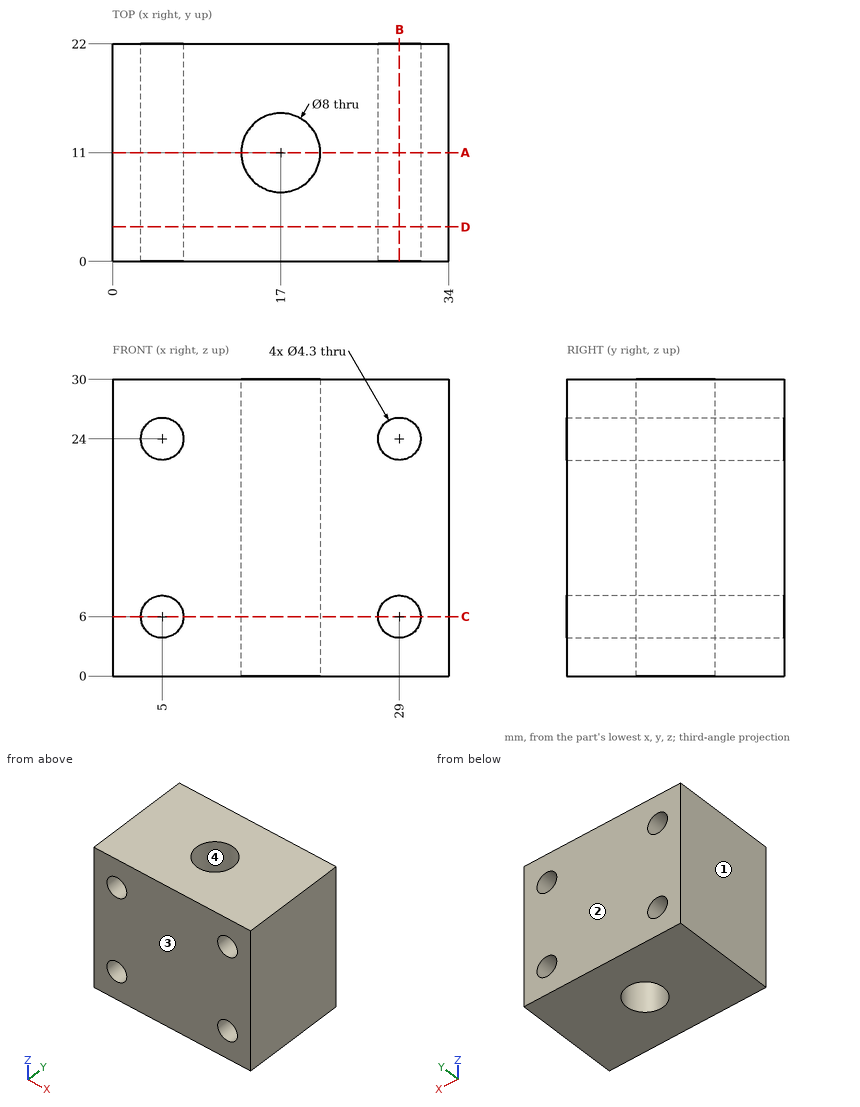
Can you work these out from the drawing? Everything is in mm from the part's minimum corner. Round coordinates to 2 decimals unless told otherwise and drop trailing zeros. Write each loop counter-clockwise with the first axis right and the second up, starting at its lowest first coordinate (ties: lowest second). Pieces come first, ordered by that corner, then holes.
1. Suppose I cut it at C-C (z = 6). List the corners of the cut face in (x, y) for me.
2. Will this pin go through, and if not, where does the flat tip stop? pin 1 Ø3.5 at (x, z) = (29, 24) entering from +Y.
3. Suppose I cut it at A-A (y = 11). List the corners of the cut face in (x, z) for me.
4. Suppose I cut it at D-D (y = 3.5). List the corners of the cut face in (x, z) for me.
5. Suppose I cut it at B-B (x = 29). List the corners of the cut face in (y, z) for me, and give its area (3 significant figures).
6. If we mould it in two halves opening along Y, with no side actions, what happens to the marked faces 1, 2, 3 and 4? For each: released by +Y, released by -Y, zero draft, split by the parting line, or undercut.
7. I need wall thicknesses on L1, parallel to Z at x = 5, y = 4.5; L2, parallel to Z at x = 6, y = 9.25; L3, parallel to Y at x = 19.5, z = 24.5. Which ranges of each line are inside material? Lowest first, please.
Answer sheet:
1. outline: (0, 0) - (2.85, 0) - (2.85, 22) - (0, 22) - close; (7.15, 0) - (26.85, 0) - (26.85, 22) - (7.15, 22) - close; (31.15, 0) - (34, 0) - (34, 22) - (31.15, 22) - close; hole circle Ø8 at (17, 11)
2. pin 1: passes through
3. outline: (0, 0) - (13, 0) - (13, 30) - (0, 30) - close; (21, 0) - (34, 0) - (34, 30) - (21, 30) - close; hole circle Ø4.3 at (5, 6); hole circle Ø4.3 at (5, 24); hole circle Ø4.3 at (29, 6); hole circle Ø4.3 at (29, 24)
4. outline: (0, 0) - (34, 0) - (34, 30) - (0, 30) - close; hole circle Ø4.3 at (5, 6); hole circle Ø4.3 at (5, 24); hole circle Ø4.3 at (29, 6); hole circle Ø4.3 at (29, 24)
5. outline: (0, 0) - (22, 0) - (22, 3.85) - (0, 3.85) - close; (0, 8.15) - (22, 8.15) - (22, 21.85) - (0, 21.85) - close; (0, 26.15) - (22, 26.15) - (22, 30) - (0, 30) - close
5. area: 471 mm2
6. face 1: zero draft
6. face 2: released by +Y
6. face 3: released by -Y
6. face 4: undercut
7. L1: z = 0 to 3.85, 8.15 to 21.85, 26.15 to 30
7. L2: z = 0 to 4.1, 7.9 to 22.1, 25.9 to 30
7. L3: y = 0 to 7.88, 14.12 to 22
